Verification items for this drawing (mm, ordinates from the low corner). A direction names the side the tool comes from. Coordinates: 2 decimals unless noted, no trailing zeros. Write each loop counter-clockwise with the first axis right and the second up, starting at its lowest first coordinate (ties: lowest second). Pieces come first, ordered by that corner, then holes. Notation, with made-up numbers: (-9.5, 70.25) -> (-5.5, 70.25) arc R31 cw to (-5.5, 108.25) -> close; hole circle Ø6 at (57, -10.5). An arc over 180 degrees is marked (long way). One line per question, with ' | ' between items.
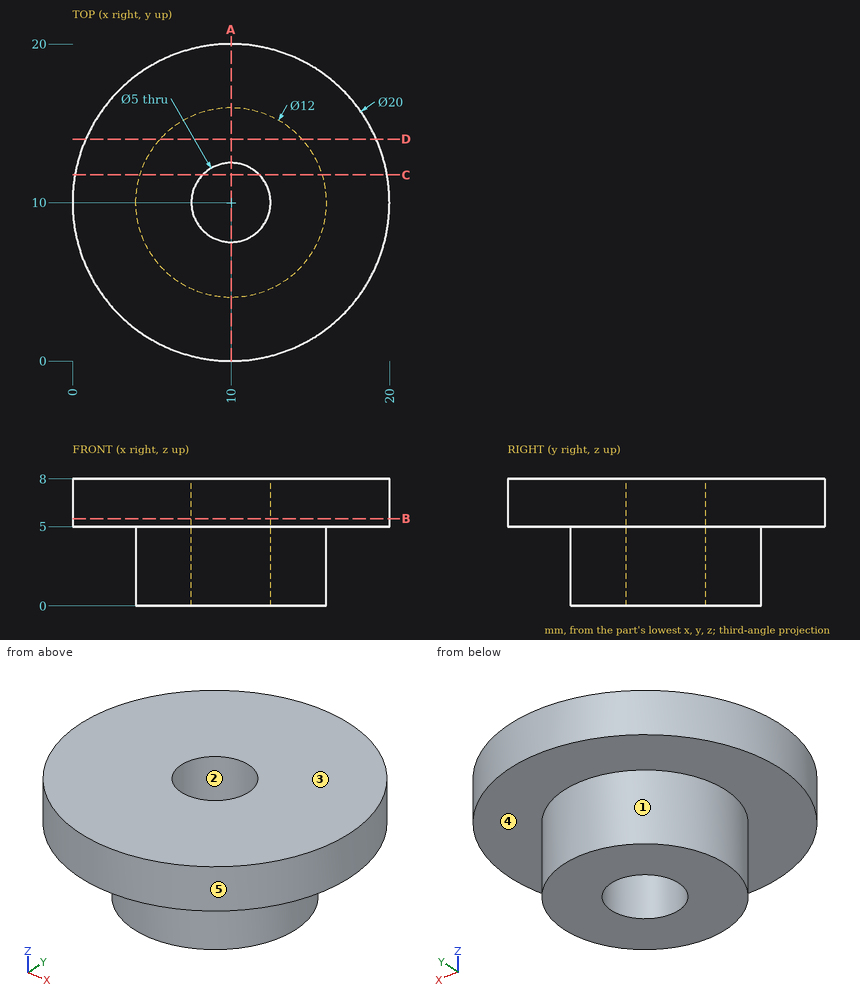
(1) Cross-section at D-D (y = 14). Record the cut outline in (x, z).
Answers below:
outline: (0.83, 5) -> (5.53, 5) -> (5.53, 0) -> (14.47, 0) -> (14.47, 5) -> (19.17, 5) -> (19.17, 8) -> (0.83, 8) -> close
(2) Tool access check on the marked faces 4 and 5. Record the directions out of +Z, -Z, +X, -X, +Y, -Y that give a thin tool (end or side, any length) a straight path to the whole face; none if there is none.
Answers below:
face 4: -Z | face 5: +Z, -Z
(3) Depth check by flat-ended pin: P1, Ø4, axis at y = 5, z = 4.5, coming from the -X side; P2, Ø4, axis at x = 10, y = 10, coming from the -Z side; P3, Ø2, axis at y = 9.5, z = 3, coming from the +X side. Enter the tip coordinate at first touch or a pass-through.
Answers below:
P1: stops at x = 0.48 | P2: passes through | P3: stops at x = 16
(4) Material ranges on line 1 (Y direction, x = 10, z = 2.25); line 2 (Y direction, x = 10, z = 6.25); line 3 (Z direction, x = 14.75, y = 14), recorded low to high.
Answers below:
line 1: y = 4 to 7.5, 12.5 to 16 | line 2: y = 0 to 7.5, 12.5 to 20 | line 3: z = 5 to 8
(5) Cross-section at B-B (z = 5.5). Record the cut outline in (x, y), plus the area to 3 significant figures.
Answers below:
outline: circle Ø20 at (10, 10); hole circle Ø5 at (10, 10) | area: 295 mm²
(6) Cross-section at A-A (x = 10). Record the cut outline in (y, z).
Answers below:
outline: (0, 5) -> (4, 5) -> (4, 0) -> (7.5, 0) -> (7.5, 8) -> (0, 8) -> close; (12.5, 0) -> (16, 0) -> (16, 5) -> (20, 5) -> (20, 8) -> (12.5, 8) -> close
(7) Cross-section at C-C (y = 11.75). Record the cut outline in (x, z).
Answers below:
outline: (0.15, 5) -> (4.26, 5) -> (4.26, 0) -> (8.21, 0) -> (8.21, 8) -> (0.15, 8) -> close; (11.79, 0) -> (15.74, 0) -> (15.74, 5) -> (19.85, 5) -> (19.85, 8) -> (11.79, 8) -> close
(8) Draft check along Y on the marked faces 1, 2 and 3. Enter one of: pulls with the +Y half, pulls with the -Y half, needs draft (parallel to the pull), parting line crosses it, or undercut.
Answers below:
face 1: parting line crosses it | face 2: undercut | face 3: needs draft
